Autodesk Inventor part; units mm, degrees
ref_plane "YZ Plane" through (0, 0, 0) normal (1, 0, 0) x (0, 1, 0)
ref_plane "XZ Plane" through (0, 0, 0) normal (0, 1, 0) x (-1, 0, 0)
ref_plane "XY Plane" through (0, 0, 0) normal (0, 0, 1) x (1, 0, 0)
sketch "Sketch1" plane through (0, 0, 0) normal (0, 0, 1) x (1, 0, 0)
  circle A0 centre (60, -12) radius 5
  line L0 (0, 0) -> (0, 90) construction
  circle A1 centre (-60, -12) radius 5
  line L1 (46, -32) -> (-46, -32)
  line L2 (-46, -32) -> (-46, -110)
  line L3 (-46, -110) -> (-81, -110)
  line L4 (-81, 90) -> (88, 90)
  line L5 (88, 90) -> (88, 190)
  line L6 (88, 190) -> (156, 190)
  line L7 (156, 190) -> (156, -110)
  line L8 (156, -110) -> (46, -110)
  line L9 (46, -110) -> (46, -32)
  line L10 (-81, -110) -> (-81, 90)
  circle A2 centre (30, 67) radius 5
  circle A3 centre (-30, 67) radius 5
  circle A4 centre (60, -58) radius 5
  circle A5 centre (-60, -58) radius 5
  circle A6 centre (-61, -85) radius 4.25
  circle A7 centre (140, -80) radius 4.25
  circle A8 centre (137, 152) radius 4.25
  circle A9 centre (-61, 40) radius 4.25
  point P0 (0, -32)
  dimension "d82" = 10
  dimension "d83" = 60
  dimension "d86" = 32
  dimension "d87" = 90
  dimension "d88" = 92
  dimension "d90" = 300
  dimension "d91" = 200
  dimension "d92" = 35
  dimension "d93" = 68
  dimension "d94" = 100
  dimension "d95" = 237
  dimension "d96" = 79
  dimension "d98" = 60
  dimension "d100" = 46
  dimension "d101" = 8.5
  dimension "d102" = 140
  dimension "d103" = 80
  dimension "d104" = 3
  dimension "d105" = 152
  dimension "d106" = 61
  dimension "d107" = 85
  dimension "d108" = 40
  dimension "d136" = 12
extrude "Extrusion1" add sketch "Sketch1" along normal blind 10
sketch "Sketch2" plane through (0, 0, 10) normal (0, 0, 1) x (1, 0, 0)
  line L0 (-81, 90) -> (88, 90)
  line L1 (-61, 90) -> (53, 90)
  line L2 (53, 90) -> (53, 30)
  line L3 (53, 30) -> (-61, 30)
  line L4 (-61, 30) -> (-61, 90)
  line L5 (-81, 90) -> (-81, -110)
  point P0 (0, 0)
  dimension "d111" = 114
  dimension "d112" = 60
  dimension "d113" = 20
extrude "Extrusion2" cut sketch "Sketch2" against normal blind 1.5
sketch "Sketch3" plane through (0, 0, 8.5) normal (0, 0, 1) x (1, 0, 0)
  circle A0 centre (-61, 40) radius 4.25
  circle A1 centre (-61, 40) radius 7
  point P0 (0, 0)
  dimension "d116" = 14
extrude "Extrusion3" cut sketch "Sketch3" along normal up to surface (1.5 mm away)
thread "Thread1"
thread "Thread2"
thread "Thread3"
thread "Thread4"
sketch "Sketch4" plane through (0, 0, 0) normal (0, 0, -1) x (-1, 0, 0)
  line L0 (-156, 190) -> (-156, -110)
  line L1 (-156, 190) -> (-90, 190)
  line L2 (-88, 190) -> (-156, 190)
  line L3 (-90, 190) -> (-90, 128)
  line L4 (-88, 90) -> (-88, 190)
  line L5 (-90, 190) -> (-28, 190) construction
  line L6 (-90, 128) -> (-156, 128)
  line L7 (-156, 128) -> (-156, 190)
  line L8 (-156, -110) -> (-46, -110)
  line L9 (-156, -110) -> (-92, -110)
  line L10 (-92, -110) -> (-92, -39.5)
  line L11 (-92, -39.5) -> (-156, -39.5)
  line L12 (81, -110) -> (81, 90)
  line L13 (46, -32) -> (46, -110)
  line L14 (81, -110) -> (46, -110)
  line L15 (46, -110) -> (46, 90)
  line L16 (81, 90) -> (-88, 90)
  point P0 (0, 0)
  dimension "d127" = 66
  dimension "d128" = 62
  dimension "d129" = 90
  dimension "d130" = 66
  dimension "d131" = 90
  dimension "d134" = 64
  dimension "d135" = 70.5
extrude "Extrusion4" cut sketch "Sketch4" against normal blind 4
properties part number "SUPPORT MAIN FRAME MOTOR-BALL SCREW-REV-B" material "Steel"
Work out the finished part from the listing and answer in its coordinate system (mm). A direction names the side the tool comes from. Round coordinates to 2 decimals unless told otherwise and drop trailing zeros. Write each loop counter-clockwise with the first axis right and the second up, starting at its lowest first coordinate (ties: lowest second). Pieces come first, ordered by that corner, then holes. Notation, with made-up numbers: (14.25, 45.25) - (52.25, 45.25) arc R23 cw to (52.25, 55.25) - close; hole circle Ø1 at (3.5, 43). An arc over 180 degrees is marked (long way). Answer in a Markdown table with one row per item. Add a question column.
1. A cutting plane is placed at C-C, the plane z = 6.25. Count the separate pieces of the cut face and the enclosed holes in it, and give its area (3 significant figures).
2. Given pin 1 (3 mm diameter, centred on x = 114.5, z = 1, fed in from -Y); pin 2 (1 mm diameter, centred on x = 8, z = 4, fed in from -Y); pin 3 (9 mm diameter, centred on x = 60, y = -12, fed in from +Z); pin 4 (10 mm diameter, centred on x = 94.5, y = 101.5, fed in from -Z), each flat-ended and moving along its own axis, determine where each tip first touches the part or whether it passes through.
3. A cutting plane is placed at D-D, the plane x = 30. Determine the outline of the cut face in (y, z).
4. The mould has two halves that part along Y. Classify faces 1 (the flat face through (122, 190, 7)), 2 (the flat face through (-46, -70, 7)), 3 (the cylindrical face through (-56.946, 38.723, 6.219)): +Y half, -Y half, draft (parallel to the pull), parting line (faces both ways), or undercut.
5. A cutting plane is placed at B-B, the plane y = 40. Determine the outline of the cut face in (x, z).
6. A cutting plane is placed at A-A, the plane x = 60. Determine the outline of the cut face in (y, z), and give its area (3 significant figures).
7. For faces 4 (the cylindrical face through (-68, 40, 9)), 5 (the flat face through (123, 159, 4)), 6 (the flat face through (46, -72, 5)), determine the directions among +Z, -Z, +X, -X, +Y, -Y from which every point of the face is accessible in a straight line to the end or side of a thin tool.
8. Find the intervals of material crossed by line 1 along Y through (x, z) = (60, 4); line 2 along X through (y, z) = (-80, 7.2); line 3 along X through (y, z) = (67, 3), in increasing order. Write a range as from..to.
Worked out:
| question | item | result |
|---|---|---|
| 1 | separate pieces | 1 |
| 1 | enclosed holes | 10 |
| 1 | area | 46,300 mm^2 |
| 2 | pin 1 | y = -39.5 |
| 2 | pin 2 | y = -32 |
| 2 | pin 3 | through |
| 2 | pin 4 | z = 0 |
| 3 | outline | (-32, 0) - (62, 0) - (62, 8.5) - (30, 8.5) - (30, 10) - (-32, 10) - close; (72, 0) - (90, 0) - (90, 8.5) - (72, 8.5) - close |
| 4 | face 1 | +Y half |
| 4 | face 2 | draft |
| 4 | face 3 | undercut |
| 5 | outline | (-81, 4) - (-65.25, 4) - (-65.25, 8.5) - (-68, 8.5) - (-68, 10) - (-81, 10) - close; (-56.75, 4) - (-46, 4) - (-46, 0) - (156, 0) - (156, 10) - (53, 10) - (53, 8.5) - (-56.75, 8.5) - close |
| 6 | outline | (-110, 0) - (-63, 0) - (-63, 10) - (-110, 10) - close; (-53, 0) - (-17, 0) - (-17, 10) - (-53, 10) - close; (-7, 0) - (90, 0) - (90, 10) - (-7, 10) - close |
| 6 | area | 1,800 mm^2 |
| 7 | face 4 | +Z |
| 7 | face 5 | -Z, +X, +Y |
| 7 | face 6 | +Z, -Z, -Y |
| 8 | line 1 | -110..-63, -53..-17, -7..90 |
| 8 | line 2 | -81..-46, 46..135.75, 144.25..156 |
| 8 | line 3 | -46..-35, -25..25, 35..156 |
